Part model, mm, in its own coordinate system. Coordinates: 2 decimals unless noted, no trailing zeros. Order: outer loops, then holes, each group sorted by start corner. A loop starts at its lowest first (then second) coordinate and runs counter-clockwise, first axis right, second up. Notation, with made-up numbers: M 7,27 L 28,27 A16 cw 28,48 Z; hole C 13.25,74 d4. An arc over 180 degrees is marked long. Answer in a Markdown table with one row per item. Add a question column.
from build123d import *

# Parameters (mm, degrees)
SKETCH_1_R               = 32.5
SKETCH_1_R_2             = 13.625
SKETCH_1_R_3             = 2
SKETCH_1_R_4             = 1.4
EXTRUDE_1_DEPTH          = 4
SKETCH_2_R               = 1
CUT_EXTRUDE_1_DEPTH      = 10
PATTERN_CIRCULAR_1_COUNT = 5


with BuildPart() as part:
    # 草图1 → 凸台-拉伸1 (new body)
    with BuildSketch(Plane.XY):
        Circle(SKETCH_1_R)
        Circle(SKETCH_1_R_2, mode=Mode.SUBTRACT)
        with Locations((0, -28)):
            Circle(SKETCH_1_R_3, mode=Mode.SUBTRACT)
        with Locations((-26.629582456, -8.652475842)):
            Circle(SKETCH_1_R_3, mode=Mode.SUBTRACT)
        with Locations((-16.457987064, 22.652475842)):
            Circle(SKETCH_1_R_3, mode=Mode.SUBTRACT)
        with Locations((16.457987064, 22.652475842)):
            Circle(SKETCH_1_R_3, mode=Mode.SUBTRACT)
        with Locations((26.629582456, -8.652475842)):
            Circle(SKETCH_1_R_3, mode=Mode.SUBTRACT)
        with Locations((-15.576309186, -21.438950351)):
            Circle(SKETCH_1_R_4, mode=Mode.SUBTRACT)
        with Locations((-25.202997682, 8.188950351)):
            Circle(SKETCH_1_R_4, mode=Mode.SUBTRACT)
        with Locations((0, 26.5)):
            Circle(SKETCH_1_R_4, mode=Mode.SUBTRACT)
        with Locations((25.202997682, 8.188950351)):
            Circle(SKETCH_1_R_4, mode=Mode.SUBTRACT)
        with Locations((15.576309186, -21.438950351)):
            Circle(SKETCH_1_R_4, mode=Mode.SUBTRACT)
    extrude(amount=EXTRUDE_1_DEPTH)

    # 草图2 → 切除-拉伸1 (cut)
    with BuildSketch(Plane.XY.offset(4)):
        with Locations((-13.625, 0)):
            Circle(SKETCH_2_R)
        with Locations((-32.49354651, 0.647638152)):
            Circle(SKETCH_2_R)
    extrude(amount=-CUT_EXTRUDE_1_DEPTH, mode=Mode.SUBTRACT)

    # 草图5 → 切除-旋转2 (revolve, cut)
    with BuildSketch(Plane(origin=(0, 0, 0), x_dir=(0, 0, -1), z_dir=(1, 0, 0)), mode=Mode.PRIVATE) as cut_revolve_2_sk:
        Polygon((-4, -28), (-1.4, -28), (-1.4, -30), (-4, -32.6), align=None)
    cut_revolve_2 = revolve(cut_revolve_2_sk.sketch.rotate(Axis((0, -28, 4), (0, 0, -1)), 270), axis=Axis((0, -28, 4), (0, 0, -1)), mode=Mode.SUBTRACT)

    # 阵列(圆周)1: 切除-旋转2 ×5 about axis
    pattern_circular_1_axis = Axis((0, 0, 0), (0, 0, 1))
    for i in range(1, PATTERN_CIRCULAR_1_COUNT):
        add(cut_revolve_2.rotate(pattern_circular_1_axis, i * 360 / PATTERN_CIRCULAR_1_COUNT), mode=Mode.SUBTRACT)


solid = part.part
(1) Slice it at B-B (x = 6). List the corners of the cut face in (y, z).
(2) Slice it at A-A (y = -28). List the corners of the cut face in (x, z), and give its area (3 significant figures).
(3) Wall check: line 1 (X direction, y = 21.5, z = 2.9); line 2 (X direction, y = 8, z = 3.75); line 3 (Y direction, x = 14.5, z = 3.85). Give the ranges that are in metal, low to high.
(4) Pull direction X, two halves, no side cores. Call faces 1 (the cylindrical face through (32.435, -2.062, 1.972)), 2 (the cylindrical face through (-14.55, 23.25, 0.69)), 3 (the flat face through (14, 0, 0)): pulls with the +X half, pulls with the -X half, needs draft (parallel to the pull), parting line crosses it, or undercut.
(5) Slice it at C-C (z = 2.45). State how many separate pieces and enclosed holes the cut face has, and give its area (3 significant figures).
(6) Drop flat-ended pins along their axis: P1, Ø6.5, axis at x = -16.46, y = 22.65, coming from the +Z side; P2, Ø1.5, axis at y = 6.5, z = 0.5, coming from the +X side; P3, Ø4.5, axis at x = 0, y = -28, coming from the +Z side. Give the stop position or say it passes through.
Computed:
| question | item | result |
|---|---|---|
| 1 | outline | M -31.94,0 L -12.23,0 L -12.23,4 L -31.94,4 Z; M 12.23,0 L 31.94,0 L 31.94,4 L 12.23,4 Z |
| 2 | outline | M -16.5,0 L -2,0 L -2,1.4 L -4.6,4 L -16.5,4 Z; M 2,0 L 16.5,0 L 16.5,4 L 4.6,4 L 2,1.4 Z |
| 2 | area | 109 mm^2 |
| 3 | line 1 | x = -24.37 to -19.76, -13.15 to 13.15, 19.76 to 24.37 |
| 3 | line 2 | x = -31.5 to -26.59, -23.82 to -11.03, 11.03 to 23.82, 26.59 to 31.5 |
| 3 | line 3 | y = -29.09 to -22.33, -20.54 to 18.66, 26.65 to 29.09 |
| 4 | face 1 | parting line crosses it |
| 4 | face 2 | undercut |
| 4 | face 3 | needs draft |
| 5 | separate pieces | 1 |
| 5 | enclosed holes | 11 |
| 5 | area | 2,560 mm^2 |
| 6 | P1 | stops at z = 2.65 |
| 6 | P2 | stops at x = 31.99 |
| 6 | P3 | stops at z = 1.65 |
